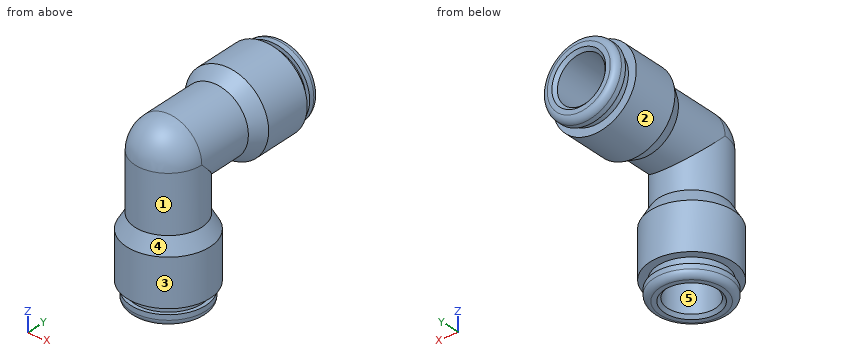
```python
from build123d import *

# Parameters (mm, degrees)
CIRPATTERN1_COUNT = 2
CIRPATTERN1_ANGLE = 90
REVOLVE2_ANGLE    = 90
CIRPATTERN2_COUNT = 2
CIRPATTERN2_ANGLE = 90


with BuildPart() as part:
    # Sketch1 → Revolve1 (revolve)
    with BuildSketch(Plane(origin=(0, 0, 0), x_dir=(0, 0, -1), z_dir=(1, 0, 0)), mode=Mode.PRIVATE) as revolve1_sk:
        with BuildLine():
            Line((15.853, 4.725), (16.488, 4.725))
            ThreePointArc((16.488, 4.725), (17.026815367, 4.501815367), (17.25, 3.963))
            Line((17.25, 3.963), (17.25, 3.381))
            Line((17.25, 3.381), (16.869, 3))
            Line((16.869, 3), (6, 3))
            Line((6, 3), (6, 2.238))
            Line((6, 2.238), (0, 2.238))
            Line((0, 2.238), (0, 4.2))
            Line((0, 4.2), (7.125, 4.2))
            Line((7.125, 4.2), (8.943653348, 5.25))
            Line((8.943653348, 5.25), (14.837, 5.25))
            Line((14.837, 5.25), (14.837, 4.2525))
            Line((14.837, 4.2525), (15.853, 4.2525))
            Line((15.853, 4.2525), (15.853, 4.725))
        make_face()
    revolve(revolve1_sk.sketch.rotate(Axis((0, 0, 0), (0, 0, -1)), 90), axis=Axis((0, 0, 0), (0, 0, -1)))


with BuildPart() as cirpattern1_1:
    # CirPattern1: pattern copy
    add(part.part.rotate(Axis((-5.775, 0, 0), (1, 0, 0)), 1 * CIRPATTERN1_ANGLE / (CIRPATTERN1_COUNT - 1)))


with BuildPart() as part_1:
    add(part.part)

    # Sketch2 → Revolve2 (revolve)
    with BuildSketch(Plane.XY):
        with BuildLine():
            Line((-4.2, 0), (-2.238, 0))
            ThreePointArc((-2.238, 0), (0, -2.238), (2.238, 0))
            Line((2.238, 0), (4.2, 0))
            ThreePointArc((4.2, 0), (0, -4.2), (-4.2, 0))
        make_face()
    revolve(axis=Axis((-4.2, 0, 0), (-1, 0, 0)), revolution_arc=REVOLVE2_ANGLE)

    # Combine1: union CirPattern1_1
    add(cirpattern1_1.part)

    # Sketch3 → Cut-Revolve1 (revolve, cut)
    with BuildSketch(Plane(origin=(0, 0, 0), x_dir=(0, 0, -1), z_dir=(1, 0, 0)), mode=Mode.PRIVATE) as cut_revolve1_sk:
        Polygon((17.25, 3.381), (16.869, 3), (6, 3), (6, 2.238), (0, 2.238), (0, 0), (17.25, 0), align=None)
    cut_revolve1 = revolve(cut_revolve1_sk.sketch.rotate(Axis((0, 0, 0), (0, 0, -1)), 90), axis=Axis((0, 0, 0), (0, 0, -1)), mode=Mode.SUBTRACT)

    # CirPattern2: Cut-Revolve1 ×2 about axis
    cirpattern2_axis = Axis((-5.775, 0, 0), (1, 0, 0))
    for i in range(1, CIRPATTERN2_COUNT):
        add(cut_revolve1.rotate(cirpattern2_axis, i * CIRPATTERN2_ANGLE / (CIRPATTERN2_COUNT - 1)), mode=Mode.SUBTRACT)


solid = part_1.part
```
Check sheet for the modelled part. Datum: model origin and axes. Units: mm. Face numbers are marked on the shaded views. A direction names the side the tool comes from. Round coordinates to 2 decimals unless told otherwise and drop trailing zeros. Loops run counter-clockwise (first coordinate to the right, second up) from the corner with the lowest first, then second, coordinate; pieces in that order, holes last. Notation, with made-up numbers: (46.5, 12.5) - (74.5, 12.5) arc R18 ccw to (74.5, 24.5) - close; hole circle Ø7 at (54, 66.5). An arc over 180 degrees is marked (long way). Write item = value, one per line. Start each with the question number.
Q1. Section check B-B (y = 8.5). Record the boundary of the cut face in (x, z).
Q2. Access from +Z, -Z, +X, -X, +Y, -Y to the whole of each face (thin tool, end or side, straight path). Record for the marked faces 1, 2 and 3.
Q3. Depth check by flat-ended pin: P1, Ø1.5, axis at x = -4, z = -2, coming from the -Y side; P2, Ø3.5, axis at x = 0, z = 0, coming from the +Y side; P3, Ø8, axis at y = 2.5, z = 2, coming from the +X side; P4, Ø3, axis at x = 2, y = -1, coming from the -Z side. Enter the tip coordinate at first touch or a pass-through.
Q4. Release check for a two-part mould opening along X. For the marked faces 4 and 5 record: pulls with the +X half, pulls with the -X half, needs draft (parallel to the pull), parting line crosses it, or undercut.
Q5. Thickness scan on L1, parallel to Z at x = 0, y = 9.25; L2, parallel to Y at x = 0, z = -1.5. Record the ranges inside material, lowest first.
Q6. Section check A-A (y = 12). Record the boundary of the cut face in (x, z), plus the area to 3 significant figures.
Derived:
q1.outline = circle Ø9.99 at (0, 0); hole circle Ø6 at (0, 0)
q2.face_1 = none
q2.face_2 = +Y
q2.face_3 = -Z
q3.P1 = -2.66
q3.P2 = -1.4
q3.P3 = 4.2
q3.P4 = -17.25
q4.face_4 = parting line crosses it
q4.face_5 = undercut
q5.L1 = -5.25 to -3, 3 to 5.25
q5.L2 = -4.2 to -2.24
q6.outline = circle Ø10.5 at (0, 0); hole circle Ø6 at (0, 0)
q6.area = 58.3 mm^2
